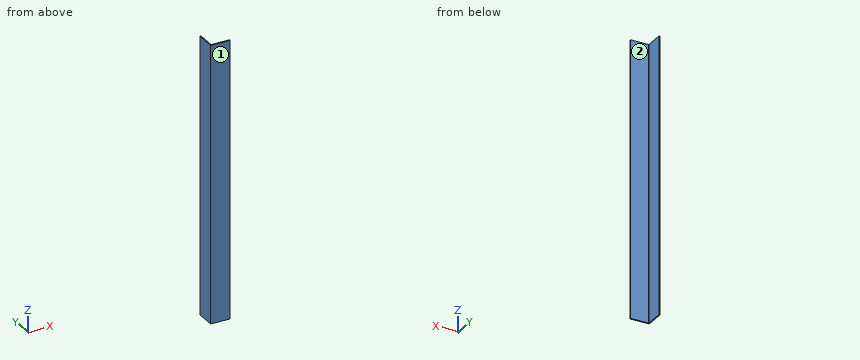
```python
from build123d import *

# Parameters (mm, degrees)
BOSS_EXTRUDE1_DEPTH = 304.8
FILLET1_R           = 0.254
CUT_EXTRUDE1_DEPTH  = 247.35


with BuildPart() as part:
    # Sketch3 → Boss-Extrude1 (new, symmetric)
    with BuildSketch(Plane.XY):
        Polygon((1.5875, 25.4), (0, 25.4), (0, 0), (25.4, 0), (25.4, 1.5875), (1.5875, 1.5875), align=None)
    extrude(amount=BOSS_EXTRUDE1_DEPTH, both=True)

    # Fillet1
    fillet1_edges = [part.edges().sort_by_distance(p)[0] for p in [
        (1.5875, 1.5875, 0),
    ]]
    fillet(fillet1_edges, radius=FILLET1_R)

    # Sketch4 → Cut-Extrude1 (cut)
    with BuildSketch(Plane(origin=(0, 0, -304.8), x_dir=(-1, 0, 0), z_dir=(0, 0, -1))):
        with BuildLine():
            Line((-1.5875, 25.4), (-1.5875, 1.8415))
            ThreePointArc((-1.5875, 1.8415), (-1.661894878, 1.661894878), (-1.8415, 1.5875))
            Line((-1.8415, 1.5875), (-25.4, 1.5875))
            Line((-25.4, 1.5875), (-25.4, 0))
            Line((-25.4, 0), (0, 0))
            Line((0, 0), (0, 25.4))
            Line((0, 25.4), (-1.5875, 25.4))
        make_face()
    extrude(amount=-CUT_EXTRUDE1_DEPTH, mode=Mode.SUBTRACT)


solid = part.part
```
Source: CAD feature listing. Evaluate the final solid. Frame: model axes, mm. Face numbers are marked on the shaded views. Give positions to 0.01 mm unless a question says otherwise; leave off trailing zeros. Write each loop counter-clockwise with the first axis right and the second up, starting at its lowest first coordinate (ties: lowest second). Pieces come first, ordered by that corner, then holes. Notation, with made-up numbers: (16.25, 13.25) - (43.25, 13.25) arc R9 ccw to (43.25, 22.25) - close; hole circle Ø7 at (33, 27). An arc over 180 degrees is marked (long way). One line per item, written item: value. Start each with the question number.
Q1. Draft query along Y for the marked faces 1 and 2. Return one class per face: +Y half, -Y half, draft (parallel to the pull), parting line (faces both ways), or undercut.
Q2. Section query A-A, the plane z = 11. Return the cut outline in (x, y).
Q3. First-contact query: pin 1 Ø10 at (y, z) = (15, 121) entering from +X; pin 2 Ø3 at (x, z) = (3.5, 61.5) entering from +Y; pin 3 Ø10 at (x, y) = (9.5, 12.5) entering from -Z. Flat tips, straight axial feed; report the tip coordinate or a pass-through.
Q4. Material intervals for probe 1 along X at (y, z) = (2.25, -16), sorted ascending. Write a range as from..to.
Q5. Section query B-B, the plane x = 20.5. Return the cut outline in (y, z).
Answer:
1. face 1: -Y half
1. face 2: +Y half
2. outline: (0, 0) - (25.4, 0) - (25.4, 1.59) - (1.84, 1.59) arc R0.25 cw to (1.59, 1.84) - (1.59, 25.4) - (0, 25.4) - close
3. pin 1: stops at x = 1.59
3. pin 2: stops at y = 1.59
3. pin 3: passes through
4. probe 1: x = 0..1.59
5. outline: (0, -57.45) - (1.59, -57.45) - (1.59, 304.8) - (0, 304.8) - close
